Geometry: final body of the model. Coordinates: model frame, mm. Give positions to 0.01 mm unless a question says otherwise; leave off trailing zeros. Write each loop counter-clockwise with the first axis right and the second up, starting at its lowest first coordinate (ties: lowest second). Pieces come first, ordered by that corner, then holes. Notation, with made-up numbers: (5.5, 62) -> (25.5, 62) arc R14 cw to (25.5, 89) -> close; hole circle Ø6 at (71, 32). An arc over 180 degrees is marked (long way). Answer in a Markdown table with one row per item. Add a question column.
from build123d import *

# Parameters (mm, degrees)
SKETCH1_R           = 72.270783293
SKETCH1_R_2         = 4
SKETCH1_R_3         = 1.050065139
SKETCH1_R_4         = 1.001019393
SKETCH1_R_5         = 0.951973647
SKETCH1_R_6         = 1.029023024
BOSS_EXTRUDE1_DEPTH = 5.08


with BuildPart() as part:
    # Sketch1 → Boss-Extrude1 (new body)
    with BuildSketch(Plane.XY):
        Circle(SKETCH1_R)
        Circle(SKETCH1_R_2, mode=Mode.SUBTRACT)
        with Locations((8, 0)):
            Circle(SKETCH1_R_3, mode=Mode.SUBTRACT)
        with Locations((0, 8)):
            Circle(SKETCH1_R_4, mode=Mode.SUBTRACT)
        with Locations((-8, 0)):
            Circle(SKETCH1_R_5, mode=Mode.SUBTRACT)
        with Locations((0, -8)):
            Circle(SKETCH1_R_6, mode=Mode.SUBTRACT)
        with BuildLine():
            Line((7.93335155, 29.556476789), (13.09319037, 48.779960759))
            ThreePointArc((13.09319037, 48.779960759), (15.685085812, 51.985178513), (19.800843937, 52.212945683))
            ThreePointArc((19.800843937, 52.212945683), (39.462982159, 39.508709884), (52.189979739, 19.86129735))
            ThreePointArc((52.189979739, 19.86129735), (51.966979092, 15.745278212), (48.764765106, 13.149672615))
            Line((48.764765106, 13.149672615), (29.547269525, 7.967574951))
            ThreePointArc((29.547269525, 7.967574951), (26.062001174, 8.275719015), (23.60265718, 10.764428592))
            ThreePointArc((23.60265718, 10.764428592), (18.33274407, 18.353987134), (10.737087643, 23.615107406))
            ThreePointArc((10.737087643, 23.615107406), (8.245531622, 26.07156763), (7.93335155, 29.556476789))
        make_face(mode=Mode.SUBTRACT)
        with BuildLine():
            Line((29.556476789, -7.93335155), (48.779960759, -13.09319037))
            ThreePointArc((48.779960759, -13.09319037), (51.985178513, -15.685085812), (52.212945683, -19.800843937))
            ThreePointArc((52.212945683, -19.800843937), (39.508709884, -39.462982159), (19.86129735, -52.189979739))
            ThreePointArc((19.86129735, -52.189979739), (15.745278212, -51.966979092), (13.149672615, -48.764765106))
            Line((13.149672615, -48.764765106), (7.967574951, -29.547269525))
            ThreePointArc((7.967574951, -29.547269525), (8.275719015, -26.062001174), (10.764428592, -23.60265718))
            ThreePointArc((10.764428592, -23.60265718), (18.353987134, -18.33274407), (23.615107406, -10.737087643))
            ThreePointArc((23.615107406, -10.737087643), (26.07156763, -8.245531622), (29.556476789, -7.93335155))
        make_face(mode=Mode.SUBTRACT)
        with BuildLine():
            Line((-7.93335155, -29.556476789), (-13.09319037, -48.779960759))
            ThreePointArc((-13.09319037, -48.779960759), (-15.685085812, -51.985178513), (-19.800843937, -52.212945683))
            ThreePointArc((-19.800843937, -52.212945683), (-39.462982159, -39.508709884), (-52.189979739, -19.86129735))
            ThreePointArc((-52.189979739, -19.86129735), (-51.966979092, -15.745278212), (-48.764765106, -13.149672615))
            Line((-48.764765106, -13.149672615), (-29.547269525, -7.967574951))
            ThreePointArc((-29.547269525, -7.967574951), (-26.062001174, -8.275719015), (-23.60265718, -10.764428592))
            ThreePointArc((-23.60265718, -10.764428592), (-18.33274407, -18.353987134), (-10.737087643, -23.615107406))
            ThreePointArc((-10.737087643, -23.615107406), (-8.245531622, -26.07156763), (-7.93335155, -29.556476789))
        make_face(mode=Mode.SUBTRACT)
        with BuildLine():
            Line((-29.556476789, 7.93335155), (-48.779960759, 13.09319037))
            ThreePointArc((-48.779960759, 13.09319037), (-51.985178513, 15.685085812), (-52.212945683, 19.800843937))
            ThreePointArc((-52.212945683, 19.800843937), (-39.508709884, 39.462982159), (-19.86129735, 52.189979739))
            ThreePointArc((-19.86129735, 52.189979739), (-15.745278212, 51.966979092), (-13.149672615, 48.764765106))
            Line((-13.149672615, 48.764765106), (-7.967574951, 29.547269525))
            ThreePointArc((-7.967574951, 29.547269525), (-8.275719015, 26.062001174), (-10.764428592, 23.60265718))
            ThreePointArc((-10.764428592, 23.60265718), (-18.353987134, 18.33274407), (-23.615107406, 10.737087643))
            ThreePointArc((-23.615107406, 10.737087643), (-26.07156763, 8.245531622), (-29.556476789, 7.93335155))
        make_face(mode=Mode.SUBTRACT)
    extrude(amount=BOSS_EXTRUDE1_DEPTH)


solid = part.part
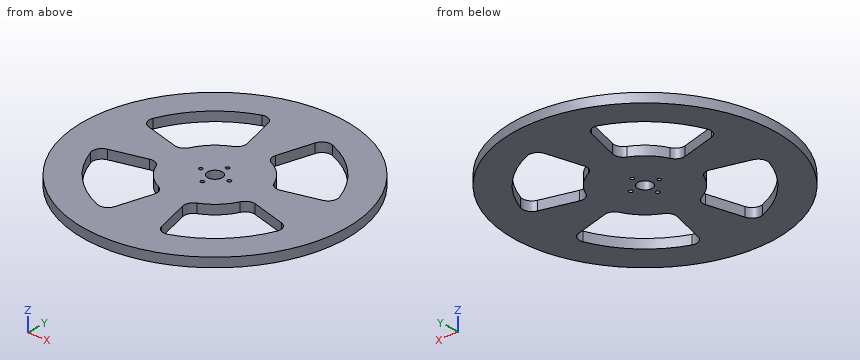
Q1. Section B-B on x = -57.5. Return loops of the section in (y, z).
Q2. Section A-A on y = -33.5. Return loops of the section in (x, z), and give its area (3 significant figures).
Q3. Contact query for flat-ended pins moving along their axis: pin 1 Ø3 at (x, y) = (0, 8) entering from -Z; pin 2 Ø1.5 at (x, z) = (-23.5, 3.5) entering from +Y; pin 3 Ø3 at (x, y) = (24, -14) entering from -Z; pin 4 Ø1 at (x, z) = (-22.5, 1.5) entering from -Y. Output: stop coordinate, or through.
Q4. Line query: probe 1 along Y at (x, z) = (0, 2); probe 2 along Y at (x, z) = (18.5, 3.25); probe 3 along X at (y, z) = (-20.5, 2.2). Output: solid intervals per line, ascending. Write a range as from..to.
Q5. Section C-C on y = -58. Return loops of the section in (x, z), and give its area (3 significant figures).
Checks:
| question | item | result |
|---|---|---|
| 1 | outline | (-43.78, 0) -> (43.78, 0) -> (43.78, 5.08) -> (-43.78, 5.08) -> close |
| 2 | outline | (-64.04, 0) -> (-44.68, 0) -> (-44.68, 5.08) -> (-64.04, 5.08) -> close; (-8.99, 0) -> (9.03, 0) -> (9.03, 5.08) -> (-8.99, 5.08) -> close; (44.68, 0) -> (64.04, 0) -> (64.04, 5.08) -> (44.68, 5.08) -> close |
| 2 | area | 288 mm^2 |
| 3 | pin 1 | z = 0 |
| 3 | pin 2 | y = 68.6 |
| 3 | pin 3 | through |
| 3 | pin 4 | y = -68.84 |
| 4 | probe 1 | -72.27..-9.03, -6.97..-4, 4..7, 9..72.27 |
| 4 | probe 2 | -69.86..-52.5, -18.19..18.19, 52.52..69.86 |
| 4 | probe 3 | -69.3..-51.94, -15.9..15.9, 51.94..69.3 |
| 5 | outline | (-43.12, 0) -> (43.12, 0) -> (43.12, 5.08) -> (-43.12, 5.08) -> close |
| 5 | area | 438 mm^2 |
